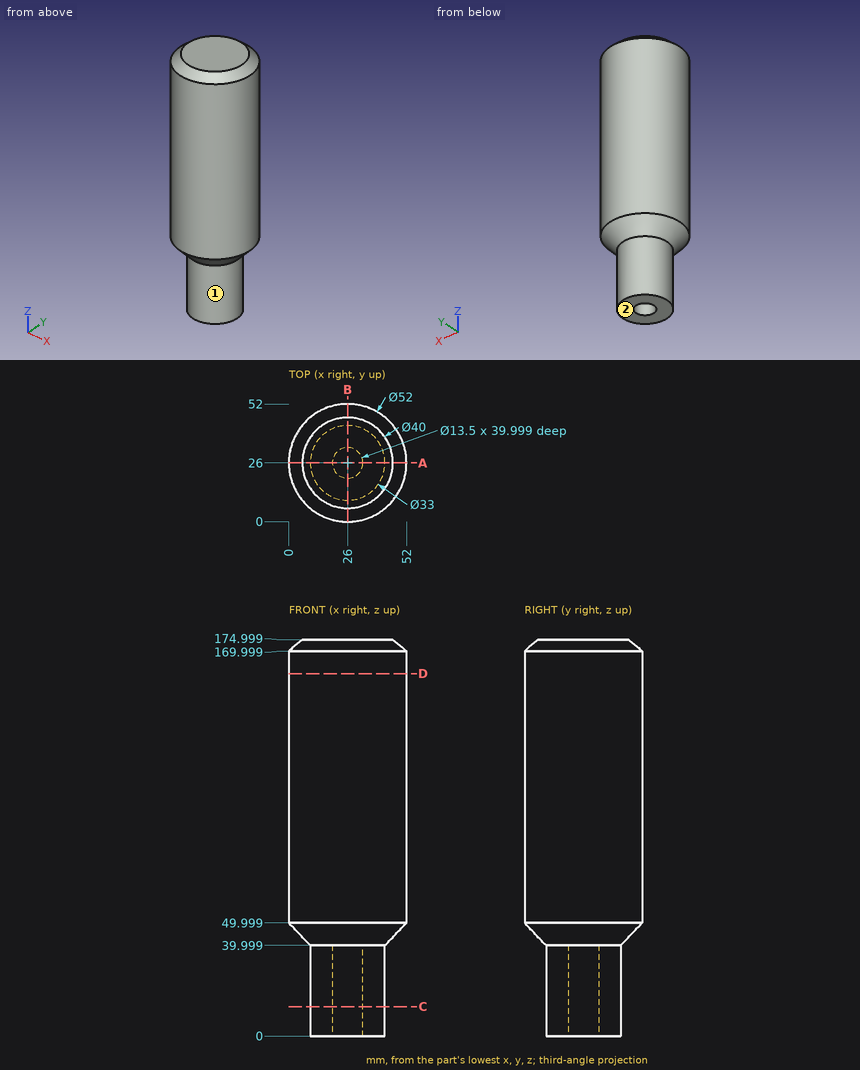
Input: dimensioned drawing with shaded views. Units: mm. Origin: part minimum x, y, z. A direction names the side the tool comes from. Coordinates: 2 decimals unless noted, no trailing zeros. Loops run counter-clockwise (first coordinate to the right, second up) from the corner with the lowest first, then second, coordinate; pieces in that order, holes last. Notation, with made-up numbers: M -19,82 L 3,82 A12 ccw 3,97 Z; hole C 52.25,25 d7. An arc over 180 degrees is marked long. Use a Markdown table: item, result. Add a question column.
1) Set-up query: the marked faces 1 and 2. Return all of +Z, -Z, +X, -X, +Y, -Y with unobstructed straight access to the full face (end or side cutting, diameter ignored); none if empty.
2) Pin query (flat end, axial travel): P1, Ø3, axis at y = 28.5, z = 56, coming from the -X side; P2, Ø10, axis at x = 32, y = 36.5, coming from the -Z side; P3, Ø4, axis at y = 46.5, z = 93, coming from the +X side; P4, Ø1.5, axis at x = 12, y = 42.5, coming from the +Z side. Return the tip coordinate at first contact, or that it passes through.
3) Section D-D, the plane z = 160. Return the cut outline in (x, y).
4) Line query: L1, parallel to Y at x = 26, z = 24; L2, parallel to Y at x = 27, z = 115; L3, parallel to Z at x = 26.5, y = 32.5. Output: solid intervals per line, ascending. Write a range as from..to.
5) Section C-C, the plane z = 13. Return the cut outline in (x, y).
6) Section A-A, the plane y = 26. Return the cut outline in (x, z), plus the area to 4 significant figures.
Answer below:
| question | item | result |
|---|---|---|
| 1 | face 1 | -Z |
| 1 | face 2 | -Z, +X, -X, +Y, -Y |
| 2 | P1 | x = 0.02 |
| 2 | P2 | z = 0 |
| 2 | P3 | x = 44.27 |
| 2 | P4 | z = 174.26 |
| 3 | outline | C 26,26 d52 |
| 4 | L1 | 9.5..19.25, 32.75..42.5 |
| 4 | L2 | 0.02..51.98 |
| 4 | L3 | 40..175 |
| 5 | outline | C 26,26 d33; hole C 26,26 d13.5 |
| 6 | outline | M 0,50 L 9.5,40 L 9.5,0 L 19.25,0 L 19.25,40 L 32.75,40 L 32.75,0 L 42.5,0 L 42.5,40 L 52,50 L 52,170 L 46,175 L 6,175 L 0,170 Z |
| 6 | area | 7,675 mm2 |
